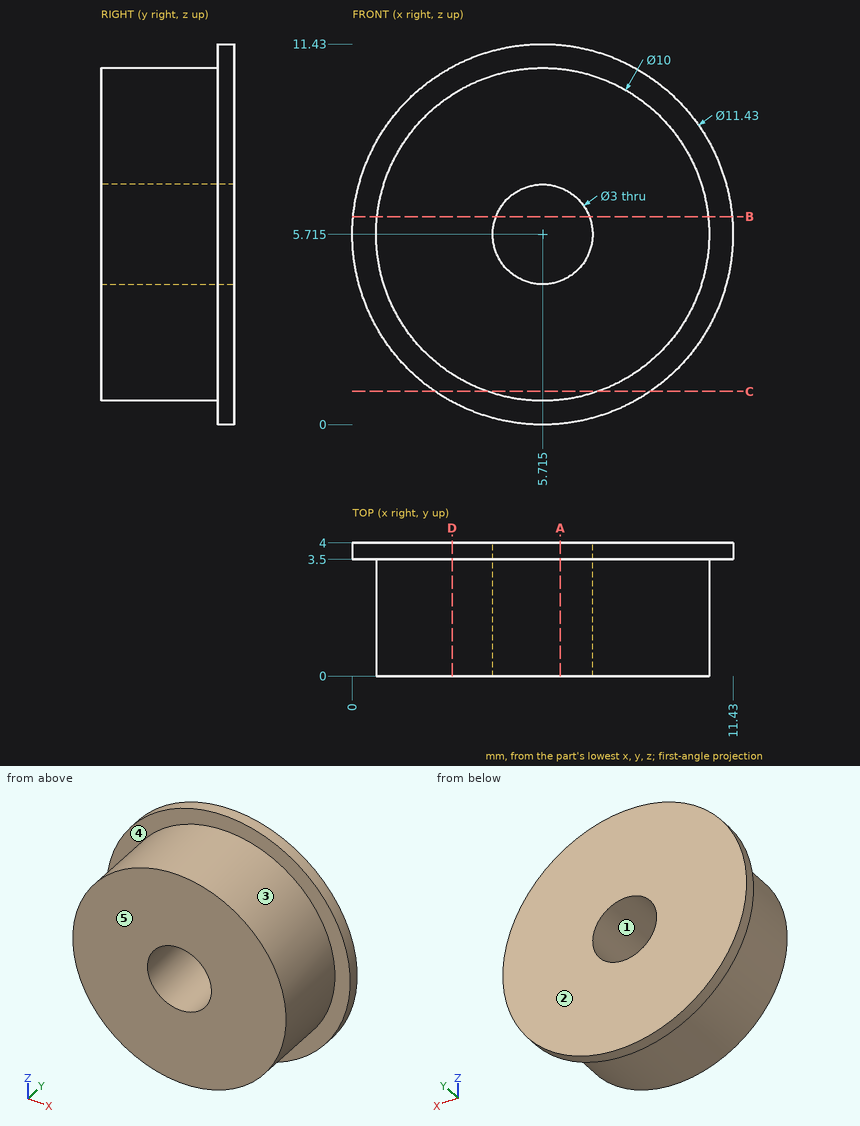
Source: three-view drawing plus pictorial views. Frame: mm from the lowest corner of the part. A direction names the side the tool comes from. Give positions to 0.01 mm unless a question says otherwise; leave off trailing zeros. Write each loop counter-clockwise with the first axis right and the second up, starting at its lowest first coordinate (ties: lowest second). Pieces come first, ordered by that corner, then holes. Notation, with made-up numbers: (84, 36.25) - (129, 36.25) arc R10 cw to (129, 47.25) - close; hole circle Ø3 at (78, 80.25). An arc over 180 degrees is marked (long way). Write item = value, one per line. Start each with the question number.
1. Access query for the marked faces 4 and 5. Directions: +Z, -Z, +X, -X, +Y, -Y. A direction counts if a zero-diameter tool reaches every point of the face in a straight line with its end or side. Return the directions, or none.
2. Section query B-B, the plane z = 6.25. Output: boundary loops of the cut face in (x, y) (1 decimal).
3. Section query D-D, the plane x = 3. Output: boundary loops of the cut face in (y, z).
4. Section query A-A, the plane x = 6.25. Output: boundary loops of the cut face in (y, z) (1 decimal).
5. Section query C-C, the plane z = 1. Output: boundary loops of the cut face in (x, y) (1 decimal).
6. First-contact query: pin 1 Ø1.5 at (x, z) = (2.5, 1.5) entering from -Y; pin 2 Ø1.5 at (y, z) = (3.5, 10) entering from -X (1 decimal); pin 3 Ø2 at (y, z) = (2, 5.5) entering from -X (1 decimal). Flat tips, straight axial feed; report the tip coordinate or a pass-through.
7. Ray query, L1, parallel to X at y = 1.7, z = 6.5 (1 decimal); L2, parallel to Z at x = 5.25, y = 0.5 (1 decimal). Return the intervals inside material, ascending.
8. Mould query, pull axis X, two halves, no side actions, for the marked faces 1, 2 and 3. Classes: released by +X, released by -X, zero draft, split by the parting line, or undercut.
Check sheet entries:
q1.face_4 = -Y
q1.face_5 = +Z, -Z, +X, -X, -Y
q2.outline = (0, 3.5) - (0.7, 3.5) - (0.7, 0) - (4.3, 0) - (4.3, 4) - (0, 4) - close; (7.1, 0) - (10.7, 0) - (10.7, 3.5) - (11.4, 3.5) - (11.4, 4) - (7.1, 4) - close
q3.outline = (0, 1.52) - (3.5, 1.52) - (3.5, 0.69) - (4, 0.69) - (4, 10.74) - (3.5, 10.74) - (3.5, 9.91) - (0, 9.91) - close
q4.outline = (0, 0.7) - (3.5, 0.7) - (3.5, 0) - (4, 0) - (4, 4.3) - (0, 4.3) - close; (0, 7.1) - (4, 7.1) - (4, 11.4) - (3.5, 11.4) - (3.5, 10.7) - (0, 10.7) - close
q5.outline = (2.5, 3.5) - (4.1, 3.5) - (4.1, 0) - (7.4, 0) - (7.4, 3.5) - (8.9, 3.5) - (8.9, 4) - (2.5, 4) - close
q6.pin_1 = 0
q6.pin_2 = 1.2
q6.pin_3 = 0.7
q7.L1 = 0.8 to 4.4, 7 to 10.7
q7.L2 = 0.7 to 4.3, 7.1 to 10.7
q8.face_1 = undercut
q8.face_2 = zero draft
q8.face_3 = split by the parting line
